The model under review builds one solid part; all positions refer to its coordinate system, in mm. Face numbers are marked on the shaded views. A direction names the side the tool comes from. Round coordinates to 2 decimals unless told otherwise and drop trailing zeros. Order: outer loops, then holes, each group sorted by start corner. A loop starts at its lowest first (then second) coordinate and runs counter-clockwise, first axis right, second up.
1) Consider section C-C (y = 3.25). Give the boundary of the cut face in (x, z).
2) Clearance check with flat-ended pins moving along their axes: P1, Ø8, axis at x = 12, z = 54, coming from the +Y side; P2, Ø1.5, axis at y = 1, z = 20, coming from the -X side; P3, Ø1.5, axis at x = 15, z = 32, coming from the -Y side. State where each tip first meets the part, or that it passes through.
3) Consider section B-B (x = 10.5). Give the boundary of the cut face in (y, z).
4) Consider section A-A (z = 10). Give the boundary of the cut face in (x, y), then the cut area to 3 significant figures.
5) To check wall thickness, follow L1, parallel to Z at x = 2.25, y = 2.75; L2, parallel to Z at x = 12, y = 0.45; L3, parallel to Z at x = 14, y = 0.4. State the ranges of each line that lie inside material, in increasing order.
6) Machinability: for the marked faces 1 and 2, which of the approach directions +Z, -Z, +X, -X, +Y, -Y give a long, thin tool a straight path to every point of the face, cutting with its end or side? Answer none if there is none.
7) Consider section D-D (x = 6.75). Give the boundary of the cut face in (y, z), then the cut area to 3 significant figures.
from build123d import *

# Parameters (mm, degrees)
BOSS_EXTRUDE1_DEPTH = 64
SKETCH2_R           = 2.499999953
CUT_EXTRUDE2_DEPTH  = 5
SKETCH3_W           = 8.000000002
SKETCH3_H           = 13
CUT_EXTRUDE3_DEPTH  = 15


with BuildPart() as part:
    # Sketch1 → Boss-Extrude1 (new body)
    with BuildSketch(Plane.XY):
        with BuildLine():
            Line((0, 0), (21.499999926, 0))
            Line((21.499999926, 0), (21.499999926, 1.4))
            Line((21.499999926, 1.4), (2.799999992, 1.4))
            ThreePointArc((2.799999992, 1.4), (-1.565247581, 6.630495138), (0, 0))
        make_face()
    extrude(amount=BOSS_EXTRUDE1_DEPTH)

    # Sketch2 → Cut-Extrude2 (cut)
    with BuildSketch(Plane(origin=(0, 0, 0), x_dir=(1, 0, 0), z_dir=(0, 1, 0))):
        with Locations(Location((11.999999876, -53.99999995, 0), (0, 0, 90))):
            Circle(SKETCH2_R)
        with Locations(Location((13.999999876, -32.000000008, 0), (0, 0, 90))):
            Circle(SKETCH2_R)
        with Locations(Location((11.999999876, -10.000000066, 0), (0, 0, 90))):
            Circle(SKETCH2_R)
    extrude(amount=CUT_EXTRUDE2_DEPTH, mode=Mode.SUBTRACT)

    # Sketch3 → Cut-Extrude3 (cut)
    with BuildSketch(Plane(origin=(0, 0, 0), x_dir=(1, 0, 0), z_dir=(0, 1, 0))):
        with Locations((1e-09, -19.499999908)):
            Rectangle(SKETCH3_W, SKETCH3_H)
        with Locations((1e-09, -44.499999908)):
            Rectangle(SKETCH3_W, SKETCH3_H)
    extrude(amount=CUT_EXTRUDE3_DEPTH, mode=Mode.SUBTRACT)


solid = part.part
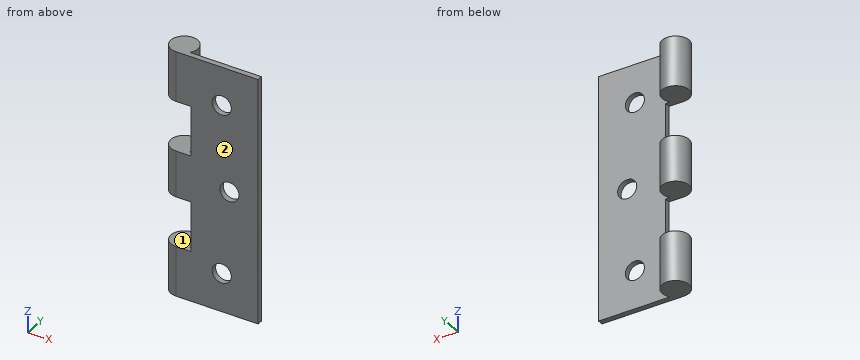
Answer below:
1. outline: (-3.49, 0) - (3.49, 0) - (3.49, 13) - (-3.49, 13) - close; (-3.49, 26) - (3.49, 26) - (3.49, 38) - (-3.49, 38) - close; (-3.49, 51) - (3.49, 51) - (3.49, 64) - (-3.49, 64) - close
2. P1: stops at y = 1.4
2. P2: stops at x = 4
2. P3: passes through
3. outline: (0, 0) - (1.4, 0) - (1.4, 8) - (0, 8) - close; (0, 12) - (1.4, 12) - (1.4, 52) - (0, 52) - close; (0, 56) - (1.4, 56) - (1.4, 64) - (0, 64) - close
4. outline: (0, 0) - (9.5, 0) - (9.5, 1.4) - (2.8, 1.4) arc R3.5 ccw (long way) to start; (14.5, 0) - (21.5, 0) - (21.5, 1.4) - (14.5, 1.4) - close
4. area: 58.8 mm2
5. L1: z = 0 to 13, 26 to 38, 51 to 64
5. L2: z = 0 to 7.5, 12.5 to 30.5, 33.5 to 51.5, 56.5 to 64
5. L3: z = 0 to 8.5, 11.5 to 29.5, 34.5 to 52.5, 55.5 to 64
6. face 1: -X, +Y, -Y
6. face 2: +Z, -Z, +X, -X, -Y
7. outline: (0, 0) - (1.4, 0) - (1.4, 64) - (0, 64) - close
7. area: 89.6 mm2
